Could you check a few things on this model? Use its own coordinates, in mm. A direction names the side the tool comes from. Round coordinates to 2 decimals unless told otherwise and drop trailing zeros. Loops run counter-clockwise (first coordinate to the right, second up) from the corner with the lowest first, then second, coordinate; pieces in that order, holes last.
from build123d import *
from build123d.topology import SkipClean

# Parameters (mm, degrees)
SKETCH1_W           = 62.5
SKETCH1_H           = 45
BOSS_EXTRUDE1_DEPTH = 20
SKETCH2_W           = 37.5
SKETCH2_H           = 45
CUT_EXTRUDE1_DEPTH  = 5
SKETCH3_R           = 11.5
CUT_EXTRUDE2_DEPTH  = 2
SKETCH4_R           = 1.5
CUT_EXTRUDE3_DEPTH  = 15
CIRPATTERN1_COUNT   = 4
SKETCH5_R           = 2.75
CUT_EXTRUDE4_DEPTH  = 58.667690261
CUT_EXTRUDE7_START  = -6.5
CUT_EXTRUDE7_DEPTH  = 3
CUT_EXTRUDE8_DEPTH  = 6.5
CUT_EXTRUDE9_DEPTH  = 5.5
SKETCH11_R          = 1.375
CUT_EXTRUDE10_DEPTH = 80.569152314
FILLET1_R           = 2
SKETCH12_R          = 3.625
CUT_EXTRUDE12_DEPTH = 3
BOSS_EXTRUDE2_START = 20
BOSS_EXTRUDE2_DEPTH = 20
SKETCH14_R          = 4
CUT_EXTRUDE18_DEPTH = 2
SKETCH15_W          = 62.5
SKETCH15_H          = 45
CUT_EXTRUDE19_DEPTH = 7
SKETCH16_R          = 3.25
CUT_EXTRUDE20_DEPTH = 64.957505524
SKETCH17_R          = 1.375
CUT_EXTRUDE21_DEPTH = 79.008012512
SKETCH18_W          = 19.875
SKETCH18_H          = 4
BOSS_EXTRUDE3_DEPTH = 4
SKETCH19_R          = 3.41
SKETCH19_R_2        = 2.5
CUT_EXTRUDE22_DEPTH = 10


with BuildPart() as part:
    # Sketch1 → Boss-Extrude1 (new body)
    with BuildSketch(Plane.XY):
        with Locations((0, 22.5)):
            Rectangle(SKETCH1_W, SKETCH1_H)
    extrude(amount=BOSS_EXTRUDE1_DEPTH)

    # Sketch2 → Cut-Extrude1 (cut)
    with BuildSketch(Plane.XY.offset(20)):
        with Locations((0, 22.5)):
            Rectangle(SKETCH2_W, SKETCH2_H)
    extrude(amount=-CUT_EXTRUDE1_DEPTH, mode=Mode.SUBTRACT)

    # Sketch3 → Cut-Extrude2 (cut)
    with BuildSketch(Plane(origin=(0, 0, 0), x_dir=(-1, 0, 0), z_dir=(0, 0, -1))):
        with Locations((0, 27.5)):
            Circle(SKETCH3_R)
    extrude(amount=-CUT_EXTRUDE2_DEPTH, mode=Mode.SUBTRACT)

    # Sketch4 → Cut-Extrude3 (cut)
    with BuildSketch(Plane(origin=(0, 0, 0), x_dir=(-1, 0, 0), z_dir=(0, 0, -1))):
        with Locations((11.5, 39)):
            Circle(SKETCH4_R)
    cut_extrude3 = extrude(amount=-CUT_EXTRUDE3_DEPTH, mode=Mode.SUBTRACT)

    # CirPattern1: Cut-Extrude3 ×4 about axis
    cirpattern1_axis = Axis((0, 27.5, 0), (0, 0, 1))
    for i in range(1, CIRPATTERN1_COUNT):
        add(cut_extrude3.rotate(cirpattern1_axis, i * 360 / CIRPATTERN1_COUNT), mode=Mode.SUBTRACT)

    # Sketch5 → Cut-Extrude4 (cut, through all)
    with BuildSketch(Plane(origin=(0, 0, 2), x_dir=(-1, 0, 0), z_dir=(0, 0, -1))):
        with Locations((0, 27.5)):
            Circle(SKETCH5_R)
    extrude(amount=-CUT_EXTRUDE4_DEPTH, mode=Mode.SUBTRACT)

    # Sketch8 → Cut-Extrude7 (cut)
    with BuildSketch(Plane(origin=(0, 0, 0), x_dir=(-1, 0, 0), z_dir=(0, 0, -1)).offset(CUT_EXTRUDE7_START)):
        with BuildLine():
            Line((7.125, 0), (-7.125, 0))
            Line((-7.125, 0), (-7.125, 11.75))
            ThreePointArc((-7.125, 11.75), (-6.539213562, 13.164213562), (-5.125, 13.75))
            Line((-5.125, 13.75), (5.125, 13.75))
            ThreePointArc((5.125, 13.75), (6.539213562, 13.164213562), (7.125, 11.75))
            Line((7.125, 11.75), (7.125, 0))
        make_face()
    extrude(amount=-CUT_EXTRUDE7_DEPTH, mode=Mode.SUBTRACT)

    # Sketch9 → Cut-Extrude8 (cut)
    with BuildSketch(Plane(origin=(0, 0, 0), x_dir=(-1, 0, 0), z_dir=(0, 0, -1))):
        with BuildLine():
            Line((4.75, 7.5), (4.75, 0))
            Line((4.75, 0), (-4.75, 0))
            Line((-4.75, 0), (-4.75, 7.5))
            ThreePointArc((-4.75, 7.5), (0, 12.25), (4.75, 7.5))
        make_face()
    extrude(amount=-CUT_EXTRUDE8_DEPTH, mode=Mode.SUBTRACT)

    # Sketch10 → Cut-Extrude9 (cut)
    with BuildSketch(Plane.XY.offset(15)):
        with BuildLine():
            Line((2.575, 7.5), (2.575, 0))
            Line((2.575, 0), (-2.575, 0))
            Line((-2.575, 0), (-2.575, 7.5))
            ThreePointArc((-2.575, 7.5), (0, 10.075), (2.575, 7.5))
        make_face()
    extrude(amount=-CUT_EXTRUDE9_DEPTH, mode=Mode.SUBTRACT)

    # Sketch11 → Cut-Extrude10 (cut, through all)
    with BuildSketch(Plane(origin=(31.25, 0, 0), x_dir=(0, 0, -1), z_dir=(1, 0, 0))):
        with Locations(Location((-17.5, 2.5, 0), (0, 0, 90))):
            Circle(SKETCH11_R)
    extrude(amount=-CUT_EXTRUDE10_DEPTH, mode=Mode.SUBTRACT)

    # Fillet1
    # the kernel refuses this fillet: 2 mm, written as the material it takes off along each edge
    with BuildSketch(Plane(origin=(31.25, 0, -5), x_dir=(0, 1, 0), z_dir=(0, 0, 1)), Plane(origin=(-31.25, 0, -5), x_dir=(1, 0, 0), z_dir=(0, 0, 1))) as fillet1_piece_1:
        with BuildLine():
            CenterArc((FILLET1_R, FILLET1_R), FILLET1_R, 180, 90)
            Line((0, FILLET1_R), (0, 0))
            Line((0, 0), (FILLET1_R, 0))
        make_face()
    extrude(amount=30, mode=Mode.SUBTRACT)

    # Sketch12 → Cut-Extrude12 (cut)
    with BuildSketch(Plane(origin=(31.25, 0, 0), x_dir=(0, 0, -1), z_dir=(1, 0, 0))):
        with Locations((-17.5, 2.5)):
            Circle(SKETCH12_R)
    cut_extrude12 = extrude(amount=-CUT_EXTRUDE12_DEPTH, mode=Mode.SUBTRACT)

    # Mirror3: Cut-Extrude12 across plane
    add(cut_extrude12.mirror(Plane(origin=(0, 0, 0), x_dir=(0, 0, 1), z_dir=(1, 0, 0))), mode=Mode.SUBTRACT)

    # Sketch13 → Boss-Extrude2 (add)
    with SkipClean():  # the faces are left unmerged after this step: merging them gives an invalid solid
        with BuildSketch(Plane(origin=(0, 0, 0), x_dir=(-1, 0, 0), z_dir=(0, 0, -1)).offset(BOSS_EXTRUDE2_START)):
            with BuildLine():
                Line((17.93986046, 0), (29.25, 0))
                ThreePointArc((29.25, 0), (30.664213562, 0.585786438), (31.25, 2))
                Line((31.25, 2), (31.25, 45))
                Line((31.25, 45), (17.93986046, 45))
                Line((17.93986046, 45), (17.93986046, 0))
            make_face()
        boss_extrude2 = extrude(amount=-BOSS_EXTRUDE2_DEPTH)

    # Sketch14 → Cut-Extrude18 (cut)
    with SkipClean():  # the faces are left unmerged after this step: merging them gives an invalid solid
        with BuildSketch(Plane.ZY.offset(31.25)):
            with BuildLine():
                ThreePointArc((-20, 3.891941091), (-20.187003937, 3.207106781), (-20.25, 2.5))
                ThreePointArc((-20.25, 2.5), (-19.58802197, 0.296001514), (-17.821195336, -1.178497685))
                ThreePointArc((-17.821195336, -1.178497685), (-14.259364049, -0.969491103), (-12.281373033, 2))
                Line((-12.281373033, 2), (-20, 2))
                Line((-20, 2), (-20, 3.891941091))
            make_face()
            with BuildLine():
                ThreePointArc((-12.25, 2.5), (-15.542893219, 6.437003937), (-20, 3.891941091))
                Line((-20, 3.891941091), (-20, 2))
                Line((-20, 2), (-12.281373033, 2))
                ThreePointArc((-12.281373033, 2), (-12.257850963, 2.24950835), (-12.25, 2.5))
            make_face()
            with BuildLine():
                ThreePointArc((-17.821195336, -1.178497685), (-19.58802197, 0.296001514), (-20.25, 2.5))
                Line((-20.25, 2.5), (-20.25, -1.178497685))
                Line((-20.25, -1.178497685), (-17.821195336, -1.178497685))
            make_face()
            with Locations((-6.25, 2.5)):
                Circle(SKETCH14_R)
        cut_extrude18 = extrude(amount=-CUT_EXTRUDE18_DEPTH, mode=Mode.SUBTRACT)

    # Sketch15 → Cut-Extrude19 (cut)
    with SkipClean():  # the faces are left unmerged after this step: merging them gives an invalid solid
        with BuildSketch(Plane.XY.offset(20)):
            with Locations((0, 22.5)):
                Rectangle(SKETCH15_W, SKETCH15_H)
        extrude(amount=-CUT_EXTRUDE19_DEPTH, mode=Mode.SUBTRACT)

    # Sketch16 → Cut-Extrude20 (cut, through all)
    with SkipClean():  # the faces are left unmerged after this step: merging them gives an invalid solid
        with BuildSketch(Plane.XY.offset(13)):
            with BuildLine():
                Line((-24.625, 0), (-24.625, 4.271707107))
                ThreePointArc((-24.625, 4.271707107), (-25, 4.25), (-25.375, 4.271707107))
                Line((-25.375, 4.271707107), (-25.375, 0))
                Line((-25.375, 0), (-24.625, 0))
            make_face()
            with Locations((-25, 7.5)):
                Circle(SKETCH16_R)
        cut_extrude20 = extrude(amount=-CUT_EXTRUDE20_DEPTH, mode=Mode.SUBTRACT)

    # Mirror4: Boss-Extrude2, Cut-Extrude18, Cut-Extrude20 across plane
    with SkipClean():  # the faces are left unmerged after this step: merging them gives an invalid solid
        add(boss_extrude2.mirror(Plane(origin=(0, 0, 0), x_dir=(0, 0, 1), z_dir=(1, 0, 0))))
        add(cut_extrude18.mirror(Plane(origin=(0, 0, 0), x_dir=(0, 0, 1), z_dir=(1, 0, 0))), mode=Mode.SUBTRACT)
        add(cut_extrude20.mirror(Plane(origin=(0, 0, 0), x_dir=(0, 0, 1), z_dir=(1, 0, 0))), mode=Mode.SUBTRACT)
    add(part.part.scale(1), mode=Mode.REPLACE)  # the faces are merged on a copy

    # Sketch17 → Cut-Extrude21 (cut, through all)
    with BuildSketch(Plane.ZY.offset(29.25)):
        with Locations(Location((-6.25, 2.5, 0), (0, 0, 180))):
            Circle(SKETCH17_R)
        with Locations(Location((-16.25, 2.5, 0), (0, 0, 180))):
            Circle(SKETCH17_R)
    extrude(amount=-CUT_EXTRUDE21_DEPTH, mode=Mode.SUBTRACT)

    # Sketch18 → Boss-Extrude3 (add)
    with BuildSketch(Plane(origin=(0, 0, 0), x_dir=(-1, 0, 0), z_dir=(0, 0, -1))):
        with BuildLine():
            Line((-51.25, 45), (-31.25, 45))
            Line((-31.25, 45), (-31.25, 2))
            ThreePointArc((-31.25, 2), (-30.664213562, 0.585786438), (-29.25, 0))
            Line((-29.25, 0), (-25.375, 0))
            Line((-25.375, 0), (-25.375, -4))
            Line((-25.375, -4), (-51.25, -4))
            Line((-51.25, -4), (-51.25, 45))
        make_face()
        with BuildLine():
            Line((50.75, -4), (50.75, 45))
            Line((50.75, 45), (31.25, 45))
            Line((31.25, 45), (31.25, 2))
            ThreePointArc((31.25, 2), (30.664213562, 0.585786438), (29.25, 0))
            Line((29.25, 0), (25.375, 0))
            Line((25.375, 0), (25.375, -4))
            Line((25.375, -4), (50.75, -4))
        make_face()
        with Locations((-14.6875, -2)):
            Rectangle(SKETCH18_W, SKETCH18_H)
        with Locations((14.6875, -2)):
            Rectangle(SKETCH18_W, SKETCH18_H)
    extrude(amount=-BOSS_EXTRUDE3_DEPTH)

    # Sketch19 → Cut-Extrude22 (cut)
    with BuildSketch(Plane(origin=(0, 0, 0), x_dir=(-1, 0, 0), z_dir=(0, 0, -1))):
        with Locations((-40.25, 6)):
            Circle(SKETCH19_R)
        with Locations((39.75, 6)):
            Circle(SKETCH19_R)
        with Locations((-40.25, 35)):
            Circle(SKETCH19_R_2)
    extrude(amount=-CUT_EXTRUDE22_DEPTH, mode=Mode.SUBTRACT)


solid = part.part
Item 1: If we section it at C-C, the plane x = 40.25: Please give me the cut outline in (y, z), then the cut area to 3 significant figures.
Results list:
outline: (-4, 0) - (2.59, 0) - (2.59, 4) - (-4, 4) - close; (9.41, 0) - (32.5, 0) - (32.5, 4) - (9.41, 4) - close; (37.5, 0) - (45, 0) - (45, 4) - (37.5, 4) - close
area: 149 mm2
Item 2: For faces 1 (the flat face through (-27, 0, -10)), 2 (the flat face through (-31.25, 23, -10)), 3 (the flat face through (-2.575, 4, 11)), which set-ups out of +Z, -Z, +X, -X, +Y, -Y let a thin tool reach every point of the face, with its end or its side?
Results list:
face 1: -Z, +X, -X, -Y
face 2: -Z, -X, +Y, -Y
face 3: +Z, -Z, -Y
Item 3: We'd pull the mould along Z, two halves only. Please class faces 4 (the flat face through (15, -2, 4)), 5 (the flat face through (27, 0, 8)), 6 (the flat face through (-25, 23, -20)), 7 (the cylindrical face through (6.6, 13.1, 8)): released by +Z, released by -Z, zero draft, split by the parting line, or undercut.
Results list:
face 4: released by +Z
face 5: zero draft
face 6: released by -Z
face 7: undercut
Item 4: If we section it at D-D, the plane y = 35: Please give me the cut outline in (x, z).
Results list:
outline: (-50.75, 0) - (-31.25, 0) - (-31.25, -20) - (-17.94, -20) - (-17.94, 0) - (-8.72, 0) - (-8.72, 2) - (8.72, 2) - (8.72, 0) - (17.94, 0) - (17.94, -20) - (31.25, -20) - (31.25, 0) - (37.75, 0) - (37.75, 4) - (31.25, 4) - (31.25, 13) - (-31.25, 13) - (-31.25, 4) - (-50.75, 4) - close; (42.75, 0) - (51.25, 0) - (51.25, 4) - (42.75, 4) - close
Item 5: If we section it at B-B, the plane z = 10.5: Please give me the cut outline in (x, y) (3 decimals), then the cut area to 3 significant figures.
Results list:
outline: (-31.25, 2) arc R2 ccw to (-29.25, 0) - (-25.375, 0) - (-25.375, 4.272) arc R3.25 cw (long way) to (-24.625, 4.272) - (-24.625, 0) - (-2.575, 0) - (-2.575, 7.5) arc R2.575 cw to (2.575, 7.5) - (2.575, 0) - (24.625, 0) - (24.625, 4.272) arc R3.25 cw (long way) to (25.375, 4.272) - (25.375, 0) - (29.25, 0) arc R2 ccw to (31.25, 2) - (31.25, 45) - (-31.25, 45) - close; hole circle Ø3 at (-11.5, 16); hole circle Ø3 at (-11.5, 39); hole circle Ø5.5 at (0, 27.5); hole circle Ø3 at (11.5, 16); hole circle Ø3 at (11.5, 39)
area: 2,640 mm2
Item 6: If I drill on line 1 along X through (y, z) = (7.5, 6); line 2 along Y through (x, z) = (40, 1); line 3 along Z through (x, y) = (21, 2.5) (3 decimals), over which ranges is the centre line in solid material (lowest first)?
Results list:
line 1: x = -31.25 to -28.25, -21.75 to -4.75, 4.75 to 21.75, 28.25 to 31.25
line 2: y = -4 to 2.6, 9.4 to 32.51, 37.49 to 45
line 3: z = -20 to -17.625, -14.875 to -7.625, -4.875 to 13
Item 7: Will these pins go through, and if not, where does the flat tip stop? pin 1 (3.5 mm diameter, centred on y = 3, z = -7, fed in from -X); pin 2 (2 mm diameter, centred on y = 2.5, z = -16.25, fed in from -X); pin 3 (5 mm diameter, centred on y = 1.5, z = -5.5, fed in from +X); pin 4 (11 mm diameter, centred on x = 2, y = 10.5, fed in from -Z).
Results list:
pin 1: stops at x = -29.25
pin 2: passes through
pin 3: stops at x = 29.25
pin 4: stops at z = 0
Item 8: If we section it at A-A, the plane x = -19.5: Please give me the cut outline in (y, z) (3 decimals), then the cut area to 3 significant figures.
Results list:
outline: (-4, 0) - (0, 0) - (0, -20) - (45, -20) - (45, 13) - (0, 13) - (0, 4) - (-4, 4) - close; hole circle Ø2.75 at (2.5, -16.25); hole circle Ø2.75 at (2.5, -6.25)
area: 1,490 mm2
